Input: part model. Units: mm. Frame: model coordinates. Face numbers are marked on the shaded views. A direction names the side the tool comes from. Give positions to 0.01 mm unless a question says otherwise; leave off trailing zeros. Order: outer loops, then holes, each group sorted by start corner. A loop starts at its lowest first (then second) coordinate and runs counter-clockwise, first axis right, second up. Notation, with made-up numbers: (67.25, -34) - (113.25, -34) arc R21 cw to (113.25, -30) - close; hole circle Ø11 at (21, 36.5). An arc over 180 degrees is marked (long way). Answer in a Markdown table with one row per item. Add a question column.
1. Section query A-A on y = 3. Return loops of the section in (x, z).
2. Access query for the marked faces 1, 2, 3, 4 and 5. Directions: +Z, -Z, +X, -X, +Y, -Y. A direction counts if a zero-diameter tool reaches every point of the face in a straight line with its end or side. Return the directions, or none.
3. Section query C-C on x = 0. Return loops of the section in (y, z), and give its area (3 significant figures).
4. Section query B-B on z = -21. Return loops of the section in (x, y).
5. Section query D-D on z = 0. Return loops of the section in (x, y), and give its area (3 significant figures).
6. Contact query for flat-ended pins moving along their axis: pin 1 (1.5 mm diameter, centred on x = 0.5, y = 3.5, fed in from -Z); pin 2 (1.5 mm diameter, centred on x = 0.5, y = 3, fed in from +Z); pin 3 (3 mm diameter, centred on y = 3, z = 13.5, fed in from +X). Output: stop coordinate, or through.
7. Ray query, line 1 (Y direction, x = 0, z = -23.7); line 2 (Z direction, x = 0, y = 3.5); line 3 (X direction, y = 4.9, z = 0). Return the intervals inside material, ascending. Write a range as [from, to].
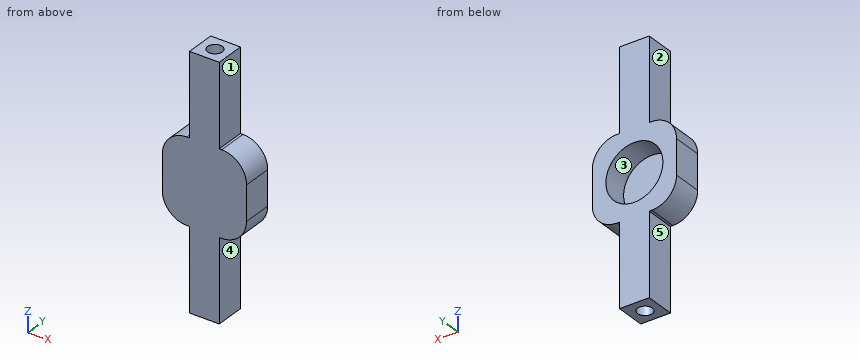
```python
from build123d import *

# Parameters (mm, degrees)
SKETCH1_R           = 5.75
BOSS_EXTRUDE1_DEPTH = 6
SKETCH8_W           = 17
SKETCH8_H           = 17
BOSS_EXTRUDE6_DEPTH = 1
FILLET1_R           = 5
SKETCH9_R           = 1.5
CUT_EXTRUDE2_DEPTH  = 5
SKETCH10_R          = 1.5
CUT_EXTRUDE3_DEPTH  = 5


with BuildPart() as part:
    # Sketch1 → Boss-Extrude1 (new body)
    with BuildSketch(Plane(origin=(0, 0, 0), x_dir=(1, 0, 0), z_dir=(0, 1, 0))):
        Polygon((8.5, 8.5), (3, 8.5), (3, 25.1), (-3, 25.1), (-3, 8.5), (-8.5, 8.5), (-8.5, -8.5), (-3, -8.5), (-3, -25.1), (3, -25.1), (3, -8.5), (8.5, -8.5), align=None)
        Circle(SKETCH1_R, mode=Mode.SUBTRACT)
    extrude(amount=BOSS_EXTRUDE1_DEPTH)

    # Sketch8 → Boss-Extrude6 (add)
    with BuildSketch(Plane.XZ):
        Rectangle(SKETCH8_W, SKETCH8_H)
    extrude(amount=-BOSS_EXTRUDE6_DEPTH)

    # Fillet1
    fillet1_edges = [part.edges().sort_by_distance(p)[0] for p in [
        (8.5, 3, -8.5),
        (-8.5, 3, -8.5),
        (-8.5, 3, 8.5),
        (8.5, 3, 8.5),
    ]]
    fillet(fillet1_edges, radius=FILLET1_R)

    # Sketch9 → Cut-Extrude2 (cut)
    with BuildSketch(Plane(origin=(0, 0, -25.1), x_dir=(-1, 0, 0), z_dir=(0, 0, -1))):
        with Locations((0, 3)):
            Circle(SKETCH9_R)
    extrude(amount=-CUT_EXTRUDE2_DEPTH, mode=Mode.SUBTRACT)

    # Sketch10 → Cut-Extrude3 (cut)
    with BuildSketch(Plane.XY.offset(25.1)):
        with Locations((0, 3)):
            Circle(SKETCH10_R)
    extrude(amount=-CUT_EXTRUDE3_DEPTH, mode=Mode.SUBTRACT)


solid = part.part
```
Answer:
| question | item | result |
|---|---|---|
| 1 | outline | (-8.5, -3.5) arc R5 ccw to (-3.5, -8.5) - (-3, -8.5) - (-3, -25.1) - (-1.5, -25.1) - (-1.5, -20.1) - (1.5, -20.1) - (1.5, -25.1) - (3, -25.1) - (3, -8.5) - (3.5, -8.5) arc R5 ccw to (8.5, -3.5) - (8.5, 3.5) arc R5 ccw to (3.5, 8.5) - (3, 8.5) - (3, 25.1) - (1.5, 25.1) - (1.5, 20.1) - (-1.5, 20.1) - (-1.5, 25.1) - (-3, 25.1) - (-3, 8.5) - (-3.5, 8.5) arc R5 ccw to (-8.5, 3.5) - close; hole circle Ø11.5 at (0, 0) |
| 2 | face 1 | +Z, +X, +Y, -Y |
| 2 | face 2 | +Z, -X, +Y, -Y |
| 2 | face 3 | +Y |
| 2 | face 4 | -Z, +X, +Y, -Y |
| 2 | face 5 | -Z, -X, +Y, -Y |
| 3 | outline | (0, -25.1) - (1.5, -25.1) - (1.5, -20.1) - (4.5, -20.1) - (4.5, -25.1) - (6, -25.1) - (6, -5.75) - (1, -5.75) - (1, 5.75) - (6, 5.75) - (6, 25.1) - (4.5, 25.1) - (4.5, 20.1) - (1.5, 20.1) - (1.5, 25.1) - (0, 25.1) - close |
| 3 | area | 214 mm² |
| 4 | outline | (-3, 0) - (3, 0) - (3, 6) - (-3, 6) - close; hole circle Ø3 at (0, 3) |
| 5 | outline | (-8.5, 0) - (8.5, 0) - (8.5, 6) - (5.75, 6) - (5.75, 1) - (-5.75, 1) - (-5.75, 6) - (-8.5, 6) - close |
| 5 | area | 44.5 mm² |
| 6 | pin 1 | stops at z = -20.1 |
| 6 | pin 2 | stops at z = 20.1 |
| 6 | pin 3 | stops at x = 3 |
| 7 | line 1 | y = [0, 1.5], [4.5, 6] |
| 7 | line 2 | z = [-20.1, -5.75], [5.75, 20.1] |
| 7 | line 3 | x = [-8.5, -5.75], [5.75, 8.5] |
